from build123d import *

# Parameters (mm, degrees)
SKETCH2_W                 = 22
SKETCH2_H                 = 22
BOSS_EXTRUDE1_DEPTH       = 6
SKETCH3_R                 = 6
CUT_EXTRUDE1_DEPTH        = 2
SKETCH4_R                 = 10.175
CUT_EXTRUDE2_DEPTH        = 4
LPATTERN1_COUNT           = 4
LPATTERN1_PITCH           = 22
LPATTERN2_COUNT           = 2
LPATTERN2_PITCH           = 22
LPATTERN2_COPY_1_SKETCH_W = 22
LPATTERN2_COPY_1_SKETCH_H = 22
LPATTERN2_COPY_1_DEPTH    = 6
LPATTERN2_COPY_2_SKETCH_W = 22
LPATTERN2_COPY_2_SKETCH_H = 22
LPATTERN2_COPY_2_DEPTH    = 6
LPATTERN2_COPY_3_SKETCH_W = 22
LPATTERN2_COPY_3_SKETCH_H = 22
LPATTERN2_COPY_3_DEPTH    = 6
LPATTERN2_COPY_4_SKETCH_R = 6
LPATTERN2_COPY_4_DEPTH    = 2
LPATTERN2_COPY_5_SKETCH_R = 6
LPATTERN2_COPY_5_DEPTH    = 2
LPATTERN2_COPY_6_SKETCH_R = 6
LPATTERN2_COPY_6_DEPTH    = 2
LPATTERN2_COPY_7_SKETCH_R = 10.175
LPATTERN2_COPY_7_DEPTH    = 4
LPATTERN2_COPY_8_SKETCH_R = 10.175
LPATTERN2_COPY_8_DEPTH    = 4
LPATTERN2_COPY_9_SKETCH_R = 10.175
LPATTERN2_COPY_9_DEPTH    = 4


with BuildPart() as part:
    # Sketch2 → Boss-Extrude1 (new body)
    with BuildSketch(Plane(origin=(0, 0, 0), x_dir=(1, 0, 0), z_dir=(0, 1, 0))):
        with Locations((11, 11)):
            Rectangle(SKETCH2_W, SKETCH2_H)
    boss_extrude1 = extrude(amount=-BOSS_EXTRUDE1_DEPTH)

    # Sketch3 → Cut-Extrude1 (cut)
    with BuildSketch(Plane(origin=(0, 0, 0), x_dir=(1, 0, 0), z_dir=(0, 1, 0))):
        with Locations(Location((11, 11.062224767, 0), (0, 0, 270))):
            Circle(SKETCH3_R)
    cut_extrude1 = extrude(amount=-CUT_EXTRUDE1_DEPTH, mode=Mode.SUBTRACT)

    # Sketch4 → Cut-Extrude2 (cut)
    with BuildSketch(Plane.XZ.offset(6)):
        with Locations(Location((11, -11.253914961, 0), (0, 0, 270))):
            Circle(SKETCH4_R)
    cut_extrude2 = extrude(amount=-CUT_EXTRUDE2_DEPTH, mode=Mode.SUBTRACT)

    # LPattern1: Boss-Extrude1, Cut-Extrude1, Cut-Extrude2 ×4
    with Locations(*[(-i * LPATTERN1_PITCH, 0, 0) for i in range(1, LPATTERN1_COUNT)]):
        add(boss_extrude1)
        add(cut_extrude1, mode=Mode.SUBTRACT)
        add(cut_extrude2, mode=Mode.SUBTRACT)

    # LPattern2: Boss-Extrude1, Cut-Extrude1, Cut-Extrude2 ×2
    with Locations(*[(0, 0, -i * LPATTERN2_PITCH) for i in range(1, LPATTERN2_COUNT)]):
        add(boss_extrude1)
        add(cut_extrude1, mode=Mode.SUBTRACT)
        add(cut_extrude2, mode=Mode.SUBTRACT)

    # LPattern2 copy 1 sketch → LPattern2 copy 1 (add)
    with BuildSketch(Plane(origin=(-22, 0, -22), x_dir=(1, 0, 0), z_dir=(0, 1, 0))):
        with Locations((11, 11)):
            Rectangle(LPATTERN2_COPY_1_SKETCH_W, LPATTERN2_COPY_1_SKETCH_H)
    extrude(amount=-LPATTERN2_COPY_1_DEPTH)

    # LPattern2 copy 2 sketch → LPattern2 copy 2 (add)
    with BuildSketch(Plane(origin=(-44, 0, -22), x_dir=(1, 0, 0), z_dir=(0, 1, 0))):
        with Locations((11, 11)):
            Rectangle(LPATTERN2_COPY_2_SKETCH_W, LPATTERN2_COPY_2_SKETCH_H)
    extrude(amount=-LPATTERN2_COPY_2_DEPTH)

    # LPattern2 copy 3 sketch → LPattern2 copy 3 (add)
    with BuildSketch(Plane(origin=(-66, 0, -22), x_dir=(1, 0, 0), z_dir=(0, 1, 0))):
        with Locations((11, 11)):
            Rectangle(LPATTERN2_COPY_3_SKETCH_W, LPATTERN2_COPY_3_SKETCH_H)
    extrude(amount=-LPATTERN2_COPY_3_DEPTH)

    # LPattern2 copy 4 sketch → LPattern2 copy 4 (cut)
    with BuildSketch(Plane(origin=(-22, 0, -22), x_dir=(1, 0, 0), z_dir=(0, 1, 0))):
        with Locations(Location((11, 11.062224767, 0), (0, 0, 270))):
            Circle(LPATTERN2_COPY_4_SKETCH_R)
    extrude(amount=-LPATTERN2_COPY_4_DEPTH, mode=Mode.SUBTRACT)

    # LPattern2 copy 5 sketch → LPattern2 copy 5 (cut)
    with BuildSketch(Plane(origin=(-44, 0, -22), x_dir=(1, 0, 0), z_dir=(0, 1, 0))):
        with Locations(Location((11, 11.062224767, 0), (0, 0, 270))):
            Circle(LPATTERN2_COPY_5_SKETCH_R)
    extrude(amount=-LPATTERN2_COPY_5_DEPTH, mode=Mode.SUBTRACT)

    # LPattern2 copy 6 sketch → LPattern2 copy 6 (cut)
    with BuildSketch(Plane(origin=(-66, 0, -22), x_dir=(1, 0, 0), z_dir=(0, 1, 0))):
        with Locations(Location((11, 11.062224767, 0), (0, 0, 270))):
            Circle(LPATTERN2_COPY_6_SKETCH_R)
    extrude(amount=-LPATTERN2_COPY_6_DEPTH, mode=Mode.SUBTRACT)

    # LPattern2 copy 7 sketch → LPattern2 copy 7 (cut)
    with BuildSketch(Plane(origin=(-22, -6, -22), x_dir=(1, 0, 0), z_dir=(0, -1, 0))):
        with Locations(Location((11, -11.253914961, 0), (0, 0, 270))):
            Circle(LPATTERN2_COPY_7_SKETCH_R)
    extrude(amount=-LPATTERN2_COPY_7_DEPTH, mode=Mode.SUBTRACT)

    # LPattern2 copy 8 sketch → LPattern2 copy 8 (cut)
    with BuildSketch(Plane(origin=(-44, -6, -22), x_dir=(1, 0, 0), z_dir=(0, -1, 0))):
        with Locations(Location((11, -11.253914961, 0), (0, 0, 270))):
            Circle(LPATTERN2_COPY_8_SKETCH_R)
    extrude(amount=-LPATTERN2_COPY_8_DEPTH, mode=Mode.SUBTRACT)

    # LPattern2 copy 9 sketch → LPattern2 copy 9 (cut)
    with BuildSketch(Plane(origin=(-66, -6, -22), x_dir=(1, 0, 0), z_dir=(0, -1, 0))):
        with Locations(Location((11, -11.253914961, 0), (0, 0, 270))):
            Circle(LPATTERN2_COPY_9_SKETCH_R)
    extrude(amount=-LPATTERN2_COPY_9_DEPTH, mode=Mode.SUBTRACT)


solid = part.part
The model under review builds one solid part; all positions refer to its coordinate system, in mm. A direction names the side the tool comes from. Give positions to 0.01 mm unless a question says otherwise; leave off trailing zeros. Order: outer loops, then holes, each group sorted by start corner. A loop starts at its lowest first (then second) coordinate and runs counter-clockwise, first axis right, second up. Notation, with made-up numbers: M 82,63.25 L 129,63.25 A27 cw 129,90.25 Z; hole C 38,62.25 d2. An arc over 180 degrees is marked long. One line per question, with ' | ' between items. Start each with the question number.
1) For faces 1 (the face through (5.14, -0.99, -12.36)), 2 (the face through (-59, -2, -16)), list the 3-axis set-ups (+Z, -Z, +X, -X, +Y, -Y) from which the entire face can be reached by the end or side of a thin tool; tool diameter is ignored.
2) Consider section C-C, the plane z = -4. Give the boundary of the cut face in (x, y).
3) Clearance check with a flat-ended pin moving along its axis: P1, Ø10, axis at x = -14, z = -9, coming from the -Y side. State where the tip first meets the part, or that it passes through.
4) Consider section D-D, the plane x = 11. Give the boundary of the cut face in (y, z), then the cut area to 3 significant figures.
5) Mouldability with a two-part tool opening along X and no side actions: class faces 3 (the face through (-22.91, -4.03, -9.93)), 4 (the face through (-66, -3, -22)), 5 (the face through (-23, -3, 0)) as pulls with the +X half, pulls with the -X half, needs draft (parallel to the pull), parting line crosses it, or undercut.
6) Consider section A-A, the plane x = -54. Give the boundary of the cut face in (y, z), then the cut area to 3 significant figures.
7) Wall thickness on L1, parallel to X at y = -1.65, z = -33; L2, parallel to Z at x = -13, y = -5.7; L3, parallel to Z at x = -62, y = -3.6: over which ranges is each line inside the solid? List them lowest first. Write a range as from..to.
8) Consider section B-B, the plane y = -1. State how many separate pieces and enclosed holes the cut face has, then the cut area to 3 significant figures.
Found:
1) face 1: +Y, -Y | face 2: -Y
2) outline: M -66,-6 L -62.14,-6 L -62.14,-2 L -47.86,-2 L -47.86,-6 L -40.14,-6 L -40.14,-2 L -25.86,-2 L -25.86,-6 L -18.14,-6 L -18.14,-2 L -3.86,-2 L -3.86,-6 L 3.86,-6 L 3.86,-2 L 18.14,-2 L 18.14,-6 L 22,-6 L 22,0 L -66,0 Z
3) P1: stops at y = -2
4) outline: M -6,-44 L 0,-44 L 0,-39.06 L -2,-39.06 L -2,-43.43 L -6,-43.43 Z; M -6,-23.08 L -2,-23.08 L -2,-27.06 L 0,-27.06 L 0,-17.06 L -2,-17.06 L -2,-21.43 L -6,-21.43 Z; M -6,-1.08 L -2,-1.08 L -2,-5.06 L 0,-5.06 L 0,0 L -6,0 Z | area: 53.2 mm²
5) face 3: undercut | face 4: pulls with the -X half | face 5: needs draft
6) outline: M -6,-44 L 0,-44 L 0,-38.98 L -2,-38.98 L -2,-43.38 L -6,-43.38 Z; M -6,-23.13 L -2,-23.13 L -2,-27.15 L 0,-27.15 L 0,-16.98 L -2,-16.98 L -2,-21.38 L -6,-21.38 Z; M -6,-1.13 L -2,-1.13 L -2,-5.15 L 0,-5.15 L 0,0 L -6,0 Z | area: 54.7 mm²
7) L1: x = -66..-61, -49..-39, -27..-17, -5..5, 17..22 | L2: z = -44..-43.23, -23.28..-21.23, -1.28..0 | L3: z = -44..-40.64, -25.87..-18.64, -3.87..0
8) separate pieces: 1 | enclosed holes: 8 | area: 2,970 mm²
